Read the model definition and answer for the solid it produces. Units are mm, in the model's axes. Face numbers are marked on the shaded views. A direction names the side the tool comes from. Give positions to 0.01 mm unless a question says otherwise; leave off trailing zeros. Loops run counter-clockwise (first coordinate to the right, second up) from the corner with the lowest first, then second, coordinate; pieces in that order, holes last.
(1) Straight lines are drawn through the part: probe 1 along Y at (x, z) = (0, 4.5); probe 2 along X at (y, z) = (-37, 4); probe 3 along Z at (x, y) = (-75.5, -29). For each, find the intervals that lie inside material, in ascending order.
(2) Each of these flat-tipped pins is pushed along its axis until it touches: P1, Ø4, axis at x = -54.5, y = -10.5, coming from the -Z side; P2, Ø3.5, axis at x = 64.95, y = -37.5, coming from the +Z side; P3, Ø8, axis at x = 39, z = -12, coming from the +Y side; P4, Ø5, axis at y = -15, z = -29.5, coming from the +X side. Where does it stop, or does it pass through?
(3) Find section C-C, the plane y = 0. Write down the section's boundary in (x, z), then the cut area to 3 significant figures.
(4) Find section D-D, the plane x = 42. Write down the section's boundary in (y, z).
(5) Which of the six approach directions +Z, -Z, +X, -X, +Y, -Y give full straight-line access (tool end or side, diameter ignored) to the marked faces 1 and 2?
(6) Find section A-A, the plane x = 0. Write down the section's boundary in (y, z).
(7) Find section B-B, the plane y = 37.5. Write down the section's boundary in (x, z), then the cut area to 3 significant figures.
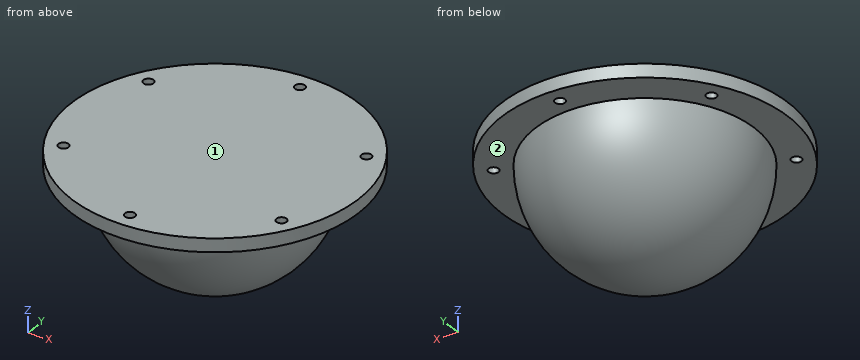
```python
from build123d import *

# Parameters (mm, degrees)
SKETCH_1_R      = 85
SKETCH_1_R_2    = 3
EXTRUDE_1_DEPTH = 8


with BuildPart() as part:
    # 草图1 → 凸台-拉伸1 (new body)
    with BuildSketch(Plane.XY):
        Circle(SKETCH_1_R)
        with Locations((0, 75)):
            Circle(SKETCH_1_R_2, mode=Mode.SUBTRACT)
        with Locations((64.951905284, 37.5)):
            Circle(SKETCH_1_R_2, mode=Mode.SUBTRACT)
        with Locations((64.951905284, -37.5)):
            Circle(SKETCH_1_R_2, mode=Mode.SUBTRACT)
        with Locations((0, -75)):
            Circle(SKETCH_1_R_2, mode=Mode.SUBTRACT)
        with Locations((-64.951905284, -37.5)):
            Circle(SKETCH_1_R_2, mode=Mode.SUBTRACT)
        with Locations((-64.951905284, 37.5)):
            Circle(SKETCH_1_R_2, mode=Mode.SUBTRACT)
    extrude(amount=EXTRUDE_1_DEPTH)

    # 草图2 → 旋转1 (revolve)
    with BuildSketch(Plane(origin=(0, 0, 0), x_dir=(1, 0, 0), z_dir=(0, 1, 0)), mode=Mode.PRIVATE) as revolve_1_sk:
        with BuildLine():
            Line((-60, 0), (-65, 0))
            ThreePointArc((-65, 0), (-45.961940777, 45.961940777), (0, 65))
            Line((0, 65), (0, 60))
            ThreePointArc((0, 60), (-42.426406871, 42.426406871), (-60, 0))
        make_face()
    revolve(revolve_1_sk.sketch.rotate(Axis((0, 0, -60), (0, 0, -1)), 180), axis=Axis((0, 0, -60), (0, 0, -1)))


solid = part.part
```
Entries:
1. probe 1: y = -85 to -78, -72 to 72, 78 to 85
1. probe 2: x = -76.52 to -67.91, -61.99 to 61.99, 67.91 to 76.52
1. probe 3: z = 0 to 8
2. P1: stops at z = -36.91
2. P2: passes through
2. P3: stops at y = 53.58
2. P4: stops at x = 57.35
3. outline: (-85, 0) - (-65, 0) arc R65 ccw to (65, 0) - (85, 0) - (85, 8) - (-85, 8) - close; hole (-60, 0) arc R60 ccw to (60, 0) - close
3. area: 2,340 mm2
4. outline: (-73.9, 0) - (-49.61, 0) arc R49.61 ccw to (49.61, 0) - (73.9, 0) - (73.9, 8) - (-73.9, 8) - close; hole (-42.85, 0) arc R42.85 ccw to (42.85, 0) - close
5. face 1: +Z, +X, -X, +Y, -Y
5. face 2: -Z
6. outline: (-85, 0) - (-78, 0) - (-78, 8) - (-85, 8) - close; (-72, 0) - (-65, 0) arc R65 ccw to (65, 0) - (72, 0) - (72, 8) - (-72, 8) - close; (78, 0) - (85, 0) - (85, 8) - (78, 8) - close; hole (-60, 0) arc R60 ccw to (60, 0) - close
7. outline: (-76.28, 0) - (-67.95, 0) - (-67.95, 8) - (-76.28, 8) - close; (-61.95, 0) - (-53.09, 0) arc R53.09 ccw to (53.09, 0) - (61.95, 0) - (61.95, 8) - (-61.95, 8) - close; (67.95, 0) - (76.28, 0) - (76.28, 8) - (67.95, 8) - close; hole (-46.84, 0) arc R46.84 ccw to (46.84, 0) - close
7. area: 2,110 mm2
